Part print with two shaded views. Sizes in mm from the minimum x, y, z corner. A direction names the side the tool comes from. Give positions to 0.01 mm unless a question says otherwise; leave off trailing zeros. Write each loop counter-clockwise with the first axis right and the second up, starting at its lowest first coordinate (ties: lowest second). Pieces come first, ordered by that corner, then holes.
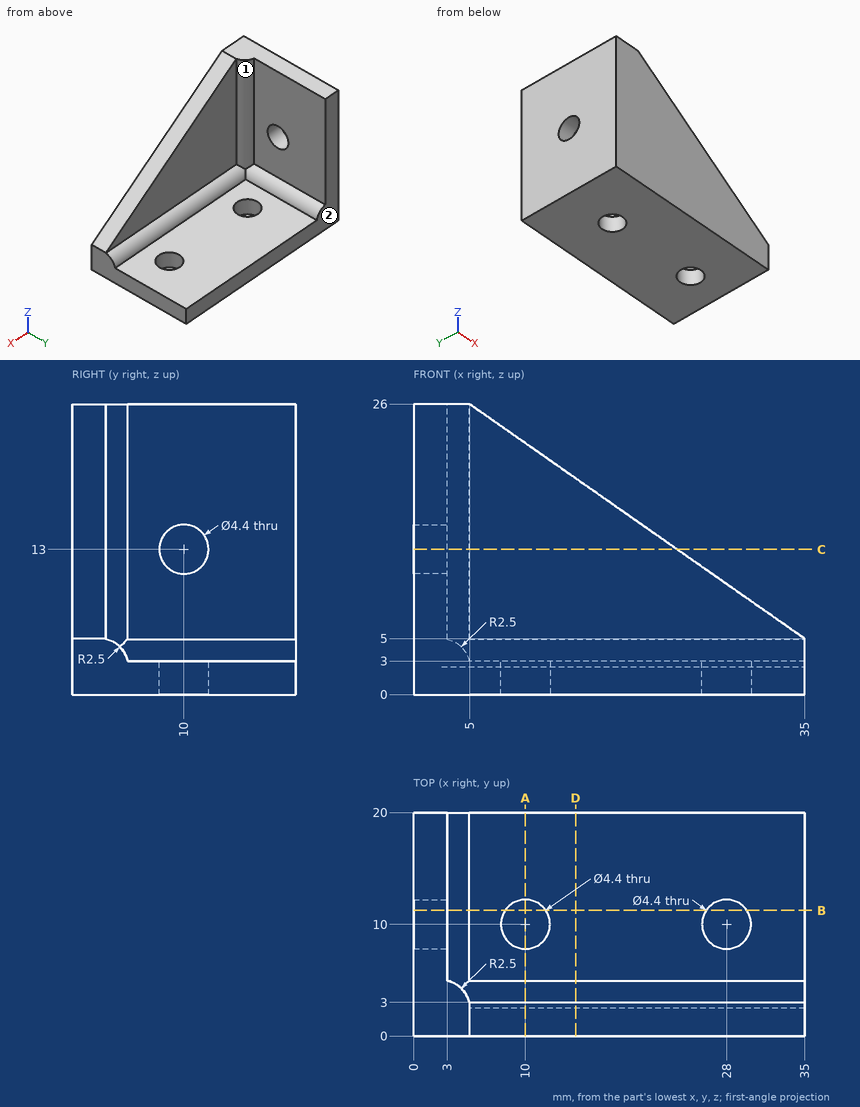
1) Drill centre lines: L1, parallel to Y at x = 28, z = 2.2; L2, parallel to Z at x = 7.5, y = 11. Where is each one in solid material? Low to high.
Check result:
L1: y = 0 to 7.8, 12.2 to 20
L2: z = 0 to 3
2) Saw through at D-D (x = 14.5). Write the cut outline in (y, z), and give its area (3 significant figures).
Check result:
outline: (0, 0) - (20, 0) - (20, 3) - (4.95, 3) arc R2.5 ccw to (3, 4.95) - (3, 19.35) - (0, 19.35) - close
area: 112 mm2
3) Saw through at B-B (y = 11.25). Write the cut outline in (x, z).
Check result:
outline: (0, 0) - (8.19, 0) - (8.19, 3) - (4.95, 3) arc R2.5 ccw to (3, 4.95) - (3, 11.19) - (0, 11.19) - close; (0, 14.81) - (3, 14.81) - (3, 26) - (0, 26) - close; (11.81, 0) - (26.19, 0) - (26.19, 3) - (11.81, 3) - close; (29.81, 0) - (35, 0) - (35, 3) - (29.81, 3) - close
4) Saw through at A-A (x = 10). Write the cut outline in (y, z).
Check result:
outline: (0, 0) - (7.8, 0) - (7.8, 3) - (4.95, 3) arc R2.5 ccw to (3, 4.95) - (3, 22.5) - (0, 22.5) - close; (12.2, 0) - (20, 0) - (20, 3) - (12.2, 3) - close
5) 3-axis set-ups, long thin cutter, end or side, ignore diameter. For the marked faces 1 and 2: which of +Z, -Z, +X, -X, +Y, -Y reach the whole face in a straight line?
Check result:
face 1: +Z, +X, +Y
face 2: +Z, -Z, +X, -X, +Y
6) Flat gauge pins, fed straight in: P1, Ø7, axis at y = 10, z = 13, coming from the +X side; P2, Ø4, axis at x = 15, y = 10.5, coming from the +Z side; P3, Ø4, axis at x = 10, y = 10, coming from the -Z side. Where does each tip first touch, or does it go through?
Check result:
P1: stops at x = 3
P2: stops at z = 3
P3: passes through
7) Saw through at C-C (z = 13). Write the cut outline in (x, y).
Check result:
outline: (0, 0) - (23.57, 0) - (23.57, 3) - (4.95, 3) arc R2.5 ccw to (3, 4.95) - (3, 7.8) - (0, 7.8) - close; (0, 12.2) - (3, 12.2) - (3, 20) - (0, 20) - close
